```python
from build123d import *

# Parameters (mm, degrees)
SKETCH_1_R          = 20
SKETCH_1_R_2        = 2.1
SKETCH_1_R_3        = 1.6
SKETCH_1_R_4        = 4
EXTRUDE_1_DEPTH     = 4
EXTRUDE_START       = -4
SKETCH_2_R          = 2.1
EXTRUDE_2_DEPTH     = 4
FILLET_1_R          = 3
CUT_EXTRUDE_START   = -4
CUT_EXTRUDE_1_DEPTH = 4
FILLET_2_R          = 4
SKETCH_4_R          = 2.15
CUT_EXTRUDE_2_DEPTH = 4


with BuildPart() as part:
    # 草图1 → 凸台-拉伸1 (new body)
    with BuildSketch(Plane(origin=(0, 0, 0), x_dir=(0, 0, -1), z_dir=(1, 0, 0))):
        Circle(SKETCH_1_R)
        with Locations((0, 16)):
            Circle(SKETCH_1_R_2, mode=Mode.SUBTRACT)
        with Locations((13.856406461, 8)):
            Circle(SKETCH_1_R_2, mode=Mode.SUBTRACT)
        with Locations((13.856406461, -8)):
            Circle(SKETCH_1_R_2, mode=Mode.SUBTRACT)
        with Locations((0, -16)):
            Circle(SKETCH_1_R_2, mode=Mode.SUBTRACT)
        with Locations((-13.856406461, -8)):
            Circle(SKETCH_1_R_2, mode=Mode.SUBTRACT)
        with Locations((-13.856406461, 8)):
            Circle(SKETCH_1_R_2, mode=Mode.SUBTRACT)
        with Locations((0, 8)):
            Circle(SKETCH_1_R_3, mode=Mode.SUBTRACT)
        with Locations((6.92820323, 4)):
            Circle(SKETCH_1_R_3, mode=Mode.SUBTRACT)
        with Locations((6.92820323, -4)):
            Circle(SKETCH_1_R_3, mode=Mode.SUBTRACT)
        with Locations((0, -8)):
            Circle(SKETCH_1_R_3, mode=Mode.SUBTRACT)
        with Locations((-6.92820323, -4)):
            Circle(SKETCH_1_R_3, mode=Mode.SUBTRACT)
        with Locations((-6.92820323, 4)):
            Circle(SKETCH_1_R_3, mode=Mode.SUBTRACT)
        Circle(SKETCH_1_R_4, mode=Mode.SUBTRACT)
    extrude(amount=EXTRUDE_1_DEPTH)

    # 草图2 → 凸台-拉伸2 (add)
    with BuildSketch(Plane(origin=(4, 0, 0), x_dir=(0, 0, -1), z_dir=(1, 0, 0)).offset(EXTRUDE_START)):
        with BuildLine():
            Line((0, -20), (50, -20))
            Line((50, -20), (72.943057454, -52.766081772))
            Line((72.943057454, -52.766081772), (122.943057454, -52.766081772))
            Line((122.943057454, -52.766081772), (122.943057454, -34.766081772))
            Line((122.943057454, -34.766081772), (82.313264364, -34.766081772))
            Line((82.313264364, -34.766081772), (57.969791834, 0))
            Line((57.969791834, 0), (6.90014553, 18.772000204))
            ThreePointArc((6.90014553, 18.772000204), (19.69060695, -3.504282802), (0, -20))
        make_face()
        with Locations((86.943057454, -43.766081772)):
            Circle(SKETCH_2_R, mode=Mode.SUBTRACT)
        with Locations((101.943057454, -43.766081772)):
            Circle(SKETCH_2_R, mode=Mode.SUBTRACT)
        with Locations((116.943057454, -43.766081772)):
            Circle(SKETCH_2_R, mode=Mode.SUBTRACT)
    extrude(amount=EXTRUDE_2_DEPTH)

    # 圆角1
    fillet_1_edges = [part.edges().sort_by_distance(p)[0] for p in [
        (2, -52.766081772, -122.943057454),
        (2, -52.766081772, -72.943057454),
        (2, -20, -50),
        (2, 0, -57.969791834),
        (2, -34.766081772, -82.313264364),
        (2, -34.766081772, -122.943057454),
    ]]
    fillet(fillet_1_edges, radius=FILLET_1_R)

    # 草图3 → 切除-拉伸1 (cut)
    with BuildSketch(Plane(origin=(4, 0, 0), x_dir=(0, 0, -1), z_dir=(1, 0, 0)).offset(CUT_EXTRUDE_START)):
        with BuildLine():
            Line((34.128214656, 3.436519896), (17.591620185, 9.514982882))
            ThreePointArc((17.591620185, 9.514982882), (19.38855853, 4.907524645), (20, 0))
            ThreePointArc((20, 0), (18.228756555, -8.228756555), (13.228756555, -15))
            Line((13.228756555, -15), (28.207788247, -15))
            Line((28.207788247, -15), (34.128214656, 3.436519896))
        make_face()
        Polygon((55.36185792, -4.368467695), (38.825263449, 1.709995291), (33.459267156, -15), (48.438298848, -15), align=None)
        with BuildLine():
            Line((58.713872022, -20.497149546), (62.15533064, -25.412061811))
            ThreePointArc((62.15533064, -25.412061811), (65.080060449, -25.927770588), (65.595769226, -23.003040779))
            Line((65.595769226, -23.003040779), (62.154310608, -18.088128513))
            ThreePointArc((62.154310608, -18.088128513), (59.229580798, -17.572419736), (58.713872022, -20.497149546))
        make_face()
        with BuildLine():
            Line((67.891095003, -33.603582254), (71.332553621, -38.51849452))
            ThreePointArc((71.332553621, -38.51849452), (74.257283431, -39.034203297), (74.772992207, -36.109473487))
            Line((74.772992207, -36.109473487), (71.331533589, -31.194561222))
            ThreePointArc((71.331533589, -31.194561222), (68.40680378, -30.678852445), (67.891095003, -33.603582254))
        make_face()
    extrude(amount=CUT_EXTRUDE_1_DEPTH, mode=Mode.SUBTRACT)

    # 圆角2
    fillet_2_edges = [part.edges().sort_by_distance(p)[0] for p in [
        (2, 1.709995291, -38.825263449),
        (2, -4.368467695, -55.36185792),
        (2, -15, -48.438298848),
        (2, -15, -33.459267156),
        (2, -15, -13.228756555),
        (2, 9.514982882, -17.591620185),
        (2, 3.436519896, -34.128214656),
        (2, -15, -28.207788247),
    ]]
    fillet(fillet_2_edges, radius=FILLET_2_R)

    # 草图4 → 切除-拉伸2 (cut)
    with BuildSketch(Plane(origin=(4, 0, 0), x_dir=(0, 0, -1), z_dir=(1, 0, 0))):
        with Locations((58.578753333, -9.586921129)):
            Circle(SKETCH_4_R)
    extrude(amount=-CUT_EXTRUDE_2_DEPTH, mode=Mode.SUBTRACT)


solid = part.part
```
Could you check a few things on this model? Use its own coordinates, in mm. A direction names the side the tool comes from. Coordinates: 2 decimals unless noted, no trailing zeros. Write each loop counter-clockwise with the first axis right and the second up, starting at its lowest first coordinate (ties: lowest second). Pieces come first, ordered by that corner, then holes. Notation, with made-up numbers: (76.25, 81.25) -> (110.25, 81.25) arc R30 ccw to (110.25, 113.25) -> close; hole circle Ø5 at (11.25, -37). An arc over 180 degrees is marked (long way). Write item = value, one per line. Start each with the question number.
(1) Will these pins go through, and if not, where does the flat tip stop? pin 1 (2 mm diameter, centred on x = 2.5, z = -68.5, fed in from +Y); pin 2 (3 mm diameter, centred on y = 4, z = 6.93, fed in from -X).
(2) Which directions (+Z, -Z, +X, -X, +Y, -Y) give clear straight access to the entire face, cutting with the end or side of a thin tool? Please do faces 1 (the face through (1.972, -17.358, -70.124)), 2 (the face through (1.97, -5.97, -36.36)).
(3) I want a section at C-C (z = -27.5). Please give me the cut outline in (x, y), plus the area to 3 significant figures.
(4) We'd pull the mould along Z, two halves only. Please class faces 3 (the face through (2, -44, -122.943)), 4 (the face through (2, -34.766, -102)), 5 (the face through (1.97, -20.58, -63.9)): released by +Z, released by -Z, zero draft, split by the parting line, or undercut.
(5) I want a section at A-A (z = -102). Please give me the cut outline in (x, y), plus the area to 3 significant figures.
(6) I want a section at B-B (x = 3). Give the number of separate pieces and of enclosed holes in the cut face, plus the area to 3 significant figures.
(7) I want a section at D-D (y = 12.5). Please give me the cut outline in (x, z), plus the area to 3 significant figures.
(8) I need wall thicknesses on line 1 (Y direction, x = 1.2, z = 0); line 2 (Y direction, x = 1.3, z = -94); line 3 (Z direction, x = 2.1, y = -42.5). Which ranges of each line are inside material? Lowest first, please. Write a range as [from, to].
Result set:
q1.pin_1 = -13.61
q1.pin_2 = through
q2.face_1 = -Z, +X, -X, +Y
q2.face_2 = +X, -X
q3.outline = (0, -20) -> (4, -20) -> (4, -14.33) -> (0, -14.33) -> close; (0, 5.87) -> (4, 5.87) -> (4, 11.2) -> (0, 11.2) -> close
q3.area = 44.0 mm2
q4.face_3 = released by -Z
q4.face_4 = zero draft
q4.face_5 = undercut
q5.outline = (0, -52.77) -> (4, -52.77) -> (4, -45.87) -> (0, -45.87) -> close; (0, -41.67) -> (4, -41.67) -> (4, -34.77) -> (0, -34.77) -> close
q5.area = 55.2 mm2
q6.separate_pieces = 1
q6.enclosed_holes = 21
q6.area = 3,090 mm2
q7.outline = (0, -23.96) -> (4, -23.96) -> (4, 15.61) -> (0, 15.61) -> close
q7.area = 158 mm2
q8.line_1 = [-20, -18.1], [-13.9, -9.6], [-6.4, -4], [4, 6.4], [9.6, 13.9], [18.1, 20]
q8.line_2 = [-52.77, -34.77]
q8.line_3 = [-122.94, -118.62], [-115.27, -103.62], [-100.27, -88.62], [-85.27, -65.75]
